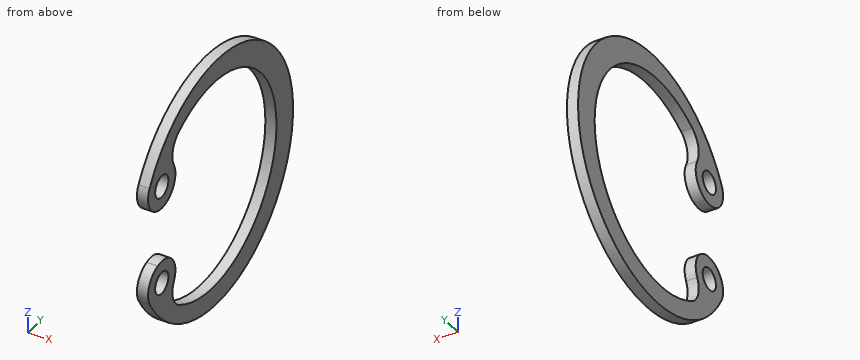
Autodesk Inventor part; units mm, degrees
ref_plane "rr_XY" through (-0.5, 0, 0) normal (1, 0, 0) x (0, 0, -1)
ref_plane "rr_YZ" through (-0.5, 0, 0) normal (0, 0, -1) x (0, 1, 0)
ref_plane "rr_ZX" through (-0.5, 0, 0) normal (0, 1, 0) x (1, 0, 0)
sketch "Sketch_3" plane through (0, 0, 0) normal (1, 0, 0) x (0, 1, 0)
  arc A0 (-10.1153, -5.4708) -> (-10.1153, 5.4708) centre (0, 0) ccw
  arc A1 (-10.1153, 5.4708) -> (-8.9159, 2.5993) centre (-8.3561, 4.5194) ccw
  line L0 (-8.9159, 2.5993) -> (-8.8563, 2.5819)
  arc A2 (-8.8563, 2.5819) -> (-6.4596, 5.4878) centre (-8.2825, 4.55) ccw
  arc A3 (-5.7223, 8.1644) -> (-6.4596, 5.4878) centre (-4.6366, 6.4255) ccw
  arc A4 (-5.7223, -8.1644) -> (-5.7223, 8.1644) centre (-0.625, 0) ccw
  arc A5 (-6.4596, -5.4878) -> (-5.7223, -8.1644) centre (-4.6366, -6.4255) ccw
  arc A6 (-6.4596, -5.4878) -> (-8.8563, -2.5819) centre (-8.2825, -4.55) ccw
  line L1 (-8.8563, -2.5819) -> (-8.9159, -2.5993)
  arc A7 (-8.9159, -2.5993) -> (-10.1153, -5.4708) centre (-8.3561, -4.5194) ccw
  circle A8 centre (-8.2825, -4.55) radius 1
  circle A9 centre (-8.2825, 4.55) radius 1
extrude "Extrusion1" add sketch "Sketch_3" along normal mid plane 1
ref_plane "rr_XY" through (-0.5, 0, 0) normal (1, 0, 0) x (0, 0, -1)
ref_plane "rr_YZ" through (-0.5, 0, 0) normal (0, 0, -1) x (0, 1, 0)
ref_plane "rr_ZX" through (-0.5, 0, 0) normal (0, 1, 0) x (1, 0, 0)
properties part number "RRING-C-INT-S-22"
Here's how the part is built. I have some questions about the finished solid (model axes, mm). Round coordinates to 2 decimals unless told otherwise and drop trailing zeros. Order: outer loops, then holes, each group sorted by start corner. A loop starts at its lowest first (then second) coordinate and runs counter-clockwise, first axis right, second up. Notation, with made-up numbers: (60, 29) -> (79, 29) arc R23 ccw to (79, 53) -> close; hole circle Ø1 at (47, 19.5). An arc over 180 degrees is marked (long way). Use a Markdown table: item, result. Add a question column.
(1) I need wall thicknesses on line 1 along Y through (x, z) = (-0.3, -5); line 2 along Z through (x, y) = (-0.4, 2.5); line 3 along Z through (x, y) = (-0.4, 2). Which ranges of each line are inside material? Lowest first, please.
(2) Suppose I cut it at C-C, the plane z = 4.55. Please give me the cut outline in (x, y).
(3) Suppose I cut it at D-D, the plane x = 0.25. Count the separate pieces of the cut face and the enclosed holes in it, and give its area (3 significant figures).
(4) Suppose I cut it at A-A, the plane z = -9.25. Please give me the cut outline in (x, y).
(5) Suppose I cut it at B-B, the plane y = 0. Please give me the cut outline in (x, z), and give its area (3 significant figures).
Verdict:
| question | item | result |
|---|---|---|
| 1 | line 1 | -10.3 to -9.18, -7.39 to -6.28, 7.6 to 10.36 |
| 1 | line 2 | -11.22 to -9.1, 9.1 to 11.22 |
| 1 | line 3 | -11.32 to -9.26, 9.26 to 11.32 |
| 2 | outline | (-0.5, -10.36) -> (0.5, -10.36) -> (0.5, -9.28) -> (-0.5, -9.28) -> close; (-0.5, -7.28) -> (0.5, -7.28) -> (0.5, -6.23) -> (-0.5, -6.23) -> close; (-0.5, 7.86) -> (0.5, 7.86) -> (0.5, 10.56) -> (-0.5, 10.56) -> close |
| 3 | separate pieces | 1 |
| 3 | enclosed holes | 2 |
| 3 | area | 129 mm2 |
| 4 | outline | (-0.5, -6.83) -> (0.5, -6.83) -> (0.5, -3.29) -> (-0.5, -3.29) -> close; (-0.5, 2.04) -> (0.5, 2.04) -> (0.5, 6.83) -> (-0.5, 6.83) -> close |
| 5 | outline | (-0.5, -11.5) -> (0.5, -11.5) -> (0.5, -9.6) -> (-0.5, -9.6) -> close; (-0.5, 9.6) -> (0.5, 9.6) -> (0.5, 11.5) -> (-0.5, 11.5) -> close |
| 5 | area | 3.79 mm2 |
